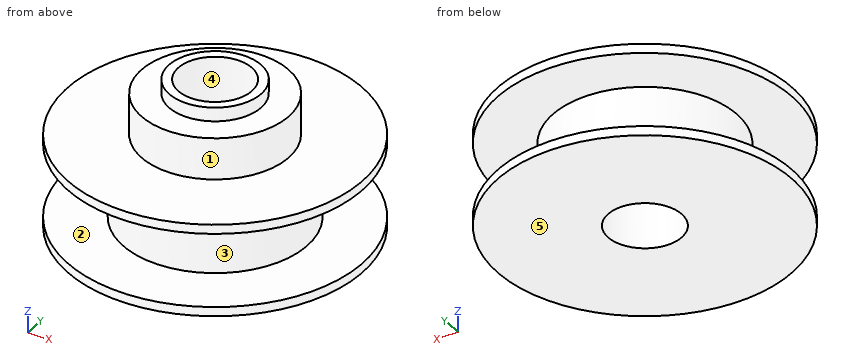
from build123d import *

# Parameters (mm, degrees)
ESQUISSE1_R             = 16
BOSS_EXTRU_1_DEPTH      = 10
ESQUISSE2_R             = 8
BOSS_EXTRU_2_DEPTH      = 6
ESQUISSE3_R             = 4
ENL_V_MAT_EXTRU_1_DEPTH = 28.712812921
ESQUISSE4_W             = 8
ESQUISSE4_H             = 6
ESQUISSE5_W             = 1.5
ESQUISSE5_H             = 3


with BuildPart() as part:
    # Esquisse1 → Boss.-Extru.1 (new body)
    with BuildSketch(Plane.XY):
        Circle(ESQUISSE1_R)
    extrude(amount=BOSS_EXTRU_1_DEPTH)

    # Esquisse2 → Boss.-Extru.2 (add)
    with BuildSketch(Plane.XY.offset(10)):
        Circle(ESQUISSE2_R)
    extrude(amount=BOSS_EXTRU_2_DEPTH)

    # Esquisse3 → Enlèv. mat.-Extru.1 (cut, through all)
    with BuildSketch(Plane.XY.offset(16)):
        Circle(ESQUISSE3_R)
    extrude(amount=-ENL_V_MAT_EXTRU_1_DEPTH, mode=Mode.SUBTRACT)

    # Esquisse4 → Enlèvement de matière-Révolution1 (revolve, cut)
    with BuildSketch(Plane(origin=(0, 0, 0), x_dir=(0, 0, -1), z_dir=(1, 0, 0)), mode=Mode.PRIVATE) as enl_vement_de_mati_re_r_volution1_sk:
        with Locations((-5, 13)):
            Rectangle(ESQUISSE4_W, ESQUISSE4_H)
    revolve(enl_vement_de_mati_re_r_volution1_sk.sketch.rotate(Axis((0, 0, 0), (0, 0, -1)), 90), axis=Axis((0, 0, 0), (0, 0, -1)), mode=Mode.SUBTRACT)

    # Esquisse5 → Enlèvement de matière-Révolution2 (revolve, cut)
    with BuildSketch(Plane(origin=(0, 0, 0), x_dir=(0, 0, -1), z_dir=(1, 0, 0)), mode=Mode.PRIVATE) as enl_vement_de_mati_re_r_volution2_sk:
        with Locations((-15.25, 6.5)):
            Rectangle(ESQUISSE5_W, ESQUISSE5_H)
    revolve(enl_vement_de_mati_re_r_volution2_sk.sketch.rotate(Axis((0, 0, 0), (0, 0, 1)), 90), axis=Axis((0, 0, 0), (0, 0, 1)), mode=Mode.SUBTRACT)


solid = part.part
Geometry: final body of the model. Coordinates: model frame, mm. Face numbers are marked on the shaded views. A direction names the side the tool comes from. Give positions to 0.01 mm unless a question says otherwise; leave off trailing zeros. Loops run counter-clockwise (first coordinate to the right, second up) from the corner with the lowest first, then second, coordinate; pieces in that order, holes last. Notation, with made-up numbers: M 37,66.25 L 78,66.25 A8 ccw 78,72.25 Z; hole C -7.75,-7 d8. An arc over 180 degrees is marked long. Put each result on its own line as item: value. Start each with the question number.
1) Access query for the marked faces 1 and 2. Directions: +Z, -Z, +X, -X, +Y, -Y. A direction counts if a zero-diameter tool reaches every point of the face in a straight line with its end or side. Return the directions, or none.
2) Contact query for flat-ended pins moving along their axis: pin 1 (13 mm diameter, centred on x = 0, y = 0, fed in from +Z); pin 2 (6 mm diameter, centred on x = 10, z = 9.5, fed in from +Y); pin 3 (3 mm diameter, centred on y = 11.5, z = 13, fed in from -X); pin 4 (2 mm diameter, centred on x = -10, y = -1.5, fed in from +Z). Output: stop coordinate, or through.
3) Cut plane A-A (x = -3). Output: boundary loops of the cut face in (y, z), then the cut area to 3 significant figures.
4) Cut plane C-C (z = 11). Output: boundary loops of the cut face in (x, y).
5) Cut plane D-D (y = 7). Output: boundary loops of the cut face in (x, z).
6) Cut plane B-B (y = 0). Output: boundary loops of the cut face in (x, z).
7) Pull-direction query (X, two-part tool) for the marked faces 3, 4 and 5; classes: pulls with the +X half, pulls with the -X half, needs draft (parallel to the pull), parting line crosses it, or undercut.
8) Ray query, line 1 along Y through (x, z) = (0, 5.5); line 2 along Z through (x, y) = (-4, 11.5); line 3 along Y through (x, z) = (0, 9.5). Return the intervals inside material, ascending.
Verdict:
1. face 1: +Z
1. face 2: none
2. pin 1: z = 16
2. pin 2: y = 14.39
2. pin 3: through
2. pin 4: z = 10
3. outline: M -15.72,0 L -2.65,0 L -2.65,16 L -4,16 L -4,14.5 L -7.42,14.5 L -7.42,10 L -15.72,10 L -15.72,9 L -9.54,9 L -9.54,1 L -15.72,1 Z; M 2.65,0 L 15.72,0 L 15.72,1 L 9.54,1 L 9.54,9 L 15.72,9 L 15.72,10 L 7.42,10 L 7.42,14.5 L 4,14.5 L 4,16 L 2.65,16 Z
3. area: 210 mm2
4. outline: C 0,0 d16; hole C 0,0 d8
5. outline: M -14.39,0 L 14.39,0 L 14.39,1 L 7.14,1 L 7.14,9 L 14.39,9 L 14.39,10 L 3.87,10 L 3.87,14.5 L -3.87,14.5 L -3.87,10 L -14.39,10 L -14.39,9 L -7.14,9 L -7.14,1 L -14.39,1 Z
6. outline: M -16,0 L -4,0 L -4,16 L -5,16 L -5,14.5 L -8,14.5 L -8,10 L -16,10 L -16,9 L -10,9 L -10,1 L -16,1 Z; M 4,0 L 16,0 L 16,1 L 10,1 L 10,9 L 16,9 L 16,10 L 8,10 L 8,14.5 L 5,14.5 L 5,16 L 4,16 Z
7. face 3: parting line crosses it
7. face 4: undercut
7. face 5: needs draft
8. line 1: -10 to -4, 4 to 10
8. line 2: 0 to 1, 9 to 10
8. line 3: -16 to -4, 4 to 16
